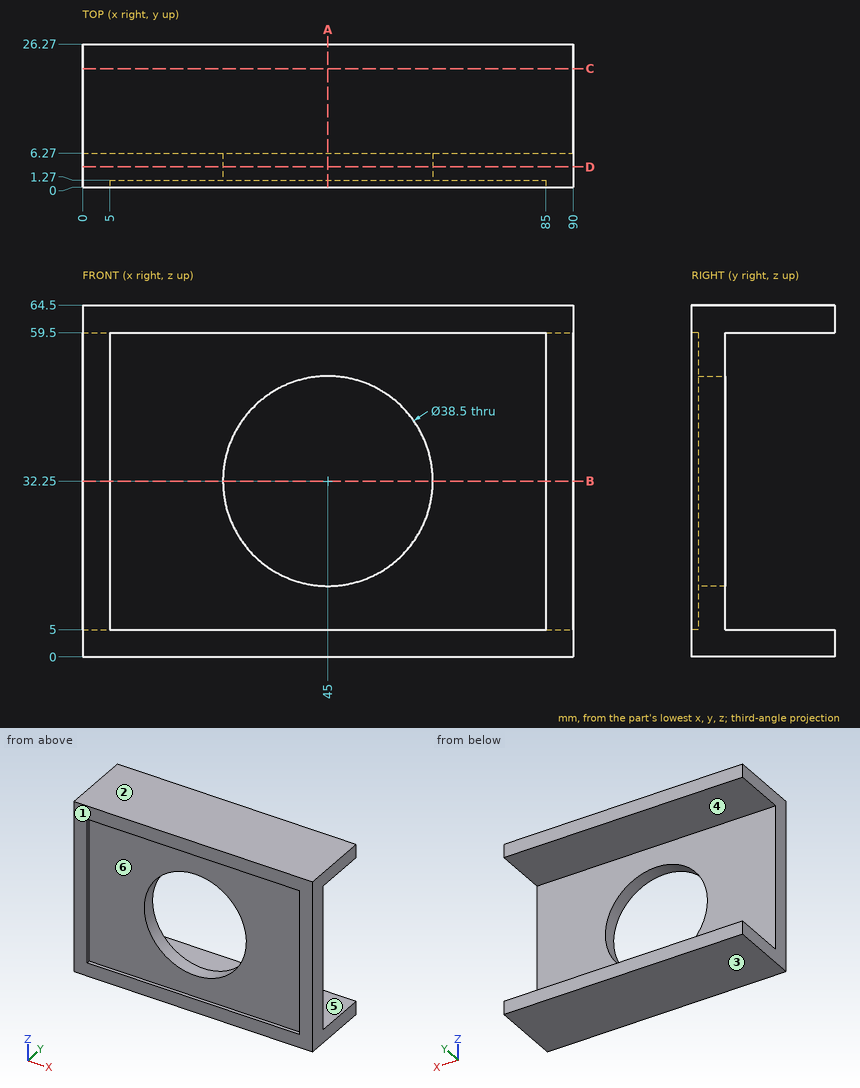
Verification items for this drawing (mm, ordinates from the low corner). A direction names the side the tool comes from. Give positions to 0.01 mm unless a question says otherwise; leave off trailing zeros. Write each loop counter-clockwise with the first axis right and the second up, starting at its lowest first coordinate (ties: lowest second). Pieces come first, ordered by that corner, then holes. Notation, with made-up numbers: (-34, 74) - (25, 74) arc R20 ccw to (25, 113) - close; hole circle Ø9 at (-32, 35.5). An arc over 180 degrees is marked (long way). Answer as a JSON object with one key per item and string values. Group by question number.
1) Depth check by flat-ended pin: P1, Ø1, axis at x = 28.5, z = 53.5, coming from the -Y side; P2, Ø2, axis at x = 61, z = 52, coming from the +Y side. Enter the tip coordinate at first touch or a pass-through.
2) Thickness scan on probe 1 along X at (y, z) = (4.5, 32.25); probe 2 along Z at (x, y) = (66.5, 17.5); probe 3 along Y at (x, z) = (29, 51). Record the ranges inside material, lowest first. Write a range as from..to.
3) Sectioned sample at A-A (x = 45). Record the cut outline in (y, z), then the cut area to 3 significant figures.
4) Access from +Z, -Z, +X, -X, +Y, -Y to the whole of each face (thin tool, end or side, straight path). Record for the marked faces 5 and 6.
5) Sectioned sample at D-D (y = 3.75). Record the cut outline in (x, z), then the cut area to 3 significant figures.
6) Release check for a two-part mould opening along Z. For the marked faces 1, 2, 3 and 4 record: pulls with the +Z half, pulls with the -Z half, needs draft (parallel to the pull), parting line crosses it, or undercut.
7) Sectioned sample at B-B (z = 32.25). Record the cut outline in (x, y).
8) Sectioned sample at C-C (y = 21.75). Record the cut outline in (x, z).
Geometry results:
{
 "1": {"P1": "stops at y = 1.27", "P2": "stops at y = 6.27"},
 "2": {"probe 1": "x = 0..25.75, 64.25..90", "probe 2": "z = 0..5, 59.5..64.5", "probe 3": "y = 1.27..6.27"},
 "3": {"outline": "(0, 0) - (26.27, 0) - (26.27, 5) - (6.27, 5) - (6.27, 13) - (1.27, 13) - (1.27, 5) - (0, 5) - close; (0, 59.5) - (1.27, 59.5) - (1.27, 51.5) - (6.27, 51.5) - (6.27, 59.5) - (26.27, 59.5) - (26.27, 64.5) - (0, 64.5) - close", "area": "343 mm^2"},
 "4": {"face 5": "+X, -X, +Y", "face 6": "-Y"},
 "5": {"outline": "(0, 0) - (90, 0) - (90, 64.5) - (0, 64.5) - close; hole circle Ø38.5 at (45, 32.25)", "area": "4,640 mm^2"},
 "6": {"face 1": "needs draft", "face 2": "pulls with the +Z half", "face 3": "pulls with the -Z half", "face 4": "undercut"},
 "7": {"outline": "(0, 0) - (5, 0) - (5, 1.27) - (25.75, 1.27) - (25.75, 6.27) - (0, 6.27) - close; (64.25, 1.27) - (85, 1.27) - (85, 0) - (90, 0) - (90, 6.27) - (64.25, 6.27) - close"},
 "8": {"outline": "(0, 0) - (90, 0) - (90, 5) - (0, 5) - close; (0, 59.5) - (90, 59.5) - (90, 64.5) - (0, 64.5) - close"}
}
